Geometry: see drawing. Coordinates: mm, zero at the bounding-box minimum. Coordinates: 2 decimals unless noted, no trailing zeros. Order: outer loops, then holes, each group sorted by start corner. A loop starts at its lowest first (then second) coordinate and runs counter-clockwise, first axis right, second up. Notation, with made-up numbers: (12, -1.5) - (22, -1.5) arc R19 ccw to (22, 14.5) - close; hole circle Ø7 at (25, 1). An arc over 180 degrees is marked (long way). Use a Markdown table: item, result. Add a question column.
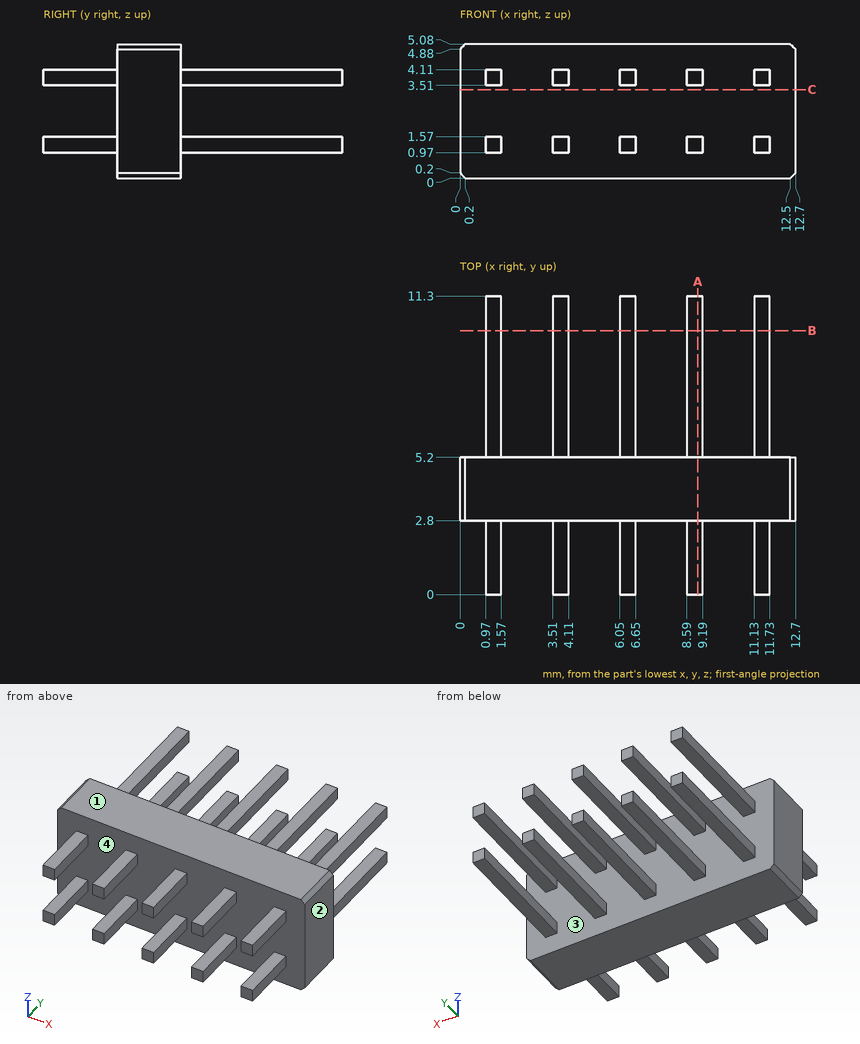
1) Section query B-B (y = 10). Give the number of separate pieces and of enclosed holes in the cut face, and give its area (3 significant figures).
2) Line query: line 1 (X direction, y = 2.5, z = 1.3); line 2 (Z direction, x = 6.5, y = 9.5); line 3 (Y direction, x = 6.5, z = 0.3). Output: solid intervals per line, ascending. Write a range as from..to.
3) Draft query along X for the marked faces 1, 2, 3 and 4. Return one class per face: released by +X, released by -X, zero draft, split by the parting line, or undercut.
4) First-contact query: pin 1 (0.5 mm diameter, centred on x = 11.5, y = 8.5, fed in from +Z); pin 2 (0.7 mm diameter, centred on x = 6.5, y = 8, fed in from -Z); pin 3 (1 mm diameter, centred on x = 4.5, y = 5, fed in from -Z); pin 4 (0.7 mm diameter, centred on y = 8.5, z = 1.5, fed in from -X). Flat tips, straight axial feed; report the tip coordinate or a pass-through.
5) Section query C-C (z = 3.35). Return the cut outline in (x, y).
6) Section query A-A (x = 9). Return the cut outline in (y, z), and give its area (3 significant figures).
From the geometry:
| question | item | result |
|---|---|---|
| 1 | separate pieces | 10 |
| 1 | enclosed holes | 0 |
| 1 | area | 3.60 mm^2 |
| 2 | line 1 | x = 0.97..1.57, 3.51..4.11, 6.05..6.65, 8.59..9.19, 11.13..11.73 |
| 2 | line 2 | z = 0.97..1.57, 3.51..4.11 |
| 2 | line 3 | y = 2.8..5.2 |
| 3 | face 1 | zero draft |
| 3 | face 2 | released by +X |
| 3 | face 3 | undercut |
| 3 | face 4 | undercut |
| 4 | pin 1 | stops at z = 4.11 |
| 4 | pin 2 | stops at z = 0.97 |
| 4 | pin 3 | stops at z = 0 |
| 4 | pin 4 | stops at x = 0.97 |
| 5 | outline | (0, 2.8) - (12.7, 2.8) - (12.7, 5.2) - (0, 5.2) - close |
| 6 | outline | (0, 0.97) - (2.8, 0.97) - (2.8, 0) - (5.2, 0) - (5.2, 0.97) - (11.3, 0.97) - (11.3, 1.57) - (5.2, 1.57) - (5.2, 3.51) - (11.3, 3.51) - (11.3, 4.11) - (5.2, 4.11) - (5.2, 5.08) - (2.8, 5.08) - (2.8, 4.11) - (0, 4.11) - (0, 3.51) - (2.8, 3.51) - (2.8, 1.57) - (0, 1.57) - close |
| 6 | area | 22.9 mm^2 |
